from build123d import *

# Parameters (mm, degrees)
SKETCH_1_R               = 2
EXTRUDE_1_DEPTH          = 74
CHAMFER_1_SIZE           = 0.5
CUT_EXTRUDE_1_DEPTH      = 75.054034326
CUT_EXTRUDE_1_DEPTH_BACK = 75.054034326
SKETCH_2_R               = 1


with BuildPart() as part:
    # 草圖1 → 填料-伸長1 (new body)
    with BuildSketch(Plane.XY):
        Circle(SKETCH_1_R)
    extrude(amount=EXTRUDE_1_DEPTH)

    # 導角1
    chamfer_1_edges = [part.edges().sort_by_distance(p)[0] for p in [
        (-2, 0, 0),
        (-2, 0, 74),
    ]]
    chamfer(chamfer_1_edges, length=CHAMFER_1_SIZE)

    # 草圖2 → 除料-伸長1 (cut, two sides: drawn at the far end of the back side and taken through both)
    with BuildSketch(Plane(origin=(0, 0, 0), x_dir=(1, 0, 0), z_dir=(0, 1, 0)).offset(-CUT_EXTRUDE_1_DEPTH_BACK)):
        with Locations(Location((0, -2, 0), (0, 0, 270))):
            Circle(SKETCH_2_R)
        with Locations(Location((0, -72, 0), (0, 0, 270))):
            Circle(SKETCH_2_R)
    extrude(amount=CUT_EXTRUDE_1_DEPTH + CUT_EXTRUDE_1_DEPTH_BACK, mode=Mode.SUBTRACT)


solid = part.part
Input: part model. Units: mm. Frame: model coordinates. Coordinates: 2 decimals unless noted, no trailing zeros. Write each loop counter-clockwise with the first axis right and the second up, starting at its lowest first coordinate (ties: lowest second). Pieces come first, ordered by that corner, then holes. Notation, with made-up numbers: M -16.75,60 L -1.75,60 A25 cw -1.75,77 Z; hole C 21.5,23 d2. An arc over 180 degrees is marked long. Answer as a JSON object with one key per item and string values. Group by question number.
(1) Section C-C on z = 60.5. Output: boundary loops of the cut face in (x, y).
(2) Section A-A on y = 0. Output: boundary loops of the cut face in (x, z), plus the area to 3 significant figures.
(3) Section D-D on z = 2. Output: boundary loops of the cut face in (x, y).
(4) Ray query, line 1 along Z through (x, y) = (0, -1); line 2 along Z through (x, y) = (0.25, -1.6); line 3 along X through (y, z) = (0.05, 2). Return the intervals inside material, ascending. Write a range as [from, to].
(5) Contact query for flat-ended pins moving along their axis: P1, Ø2, axis at x = 0.5, z = 9.5, coming from the +Y side; P2, Ø1.6, axis at x = 0, z = 72, coming from the +Y side. Output: stop coordinate, or through.
(6) Mould query, pull axis X, two halves, no side actions, for faces 1 (the face through (0, -2, 36)), 2 (the face through (0, 0, 0)), 3 (the face through (0.84, -0.03, 72.54)). Classes: pulls with the +X half, pulls with the -X half, needs draft (parallel to the pull), parting line crosses it, or undercut.
(7) Section B-B on x = 0. Output: boundary loops of the cut face in (y, z).
Result set:
{
 "1": {"outline": "C 0,0 d4"},
 "2": {"outline": "M -2,0.5 L -1.5,0 L 1.5,0 L 2,0.5 L 2,73.5 L 1.5,74 L -1.5,74 L -2,73.5 Z; hole C 0,2 d2; hole C 0,72 d2", "area": "289 mm2"},
 "3": {"outline": "M -1,-1.73 L -1,1.73 A2 ccw Z; M 1,-1.73 A2 ccw 1,1.73 Z"},
 "4": {"line 1": "z = [0, 1], [3, 71], [73, 74]", "line 2": "z = [0.12, 1.03], [2.97, 71.03], [72.97, 73.88]", "line 3": "x = [-2, -1], [1, 2]"},
 "5": {"P1": "stops at y = 2", "P2": "passes through"},
 "6": {"face 1": "parting line crosses it", "face 2": "needs draft", "face 3": "undercut"},
 "7": {"outline": "M -2,0.5 L -1.5,0 L 1.5,0 L 2,0.5 L 2,1 L -2,1 Z; M -2,3 L 2,3 L 2,71 L -2,71 Z; M -2,73 L 2,73 L 2,73.5 L 1.5,74 L -1.5,74 L -2,73.5 Z"}
}
